Build history of the part. All positions in model axes, mm. Face numbers are marked on the shaded views. A direction names the side the tool comes from. Give positions to 0.01 mm unless a question says otherwise; leave off trailing zeros. Write each loop counter-clockwise with the first axis right and the second up, starting at its lowest first coordinate (ties: lowest second). Pieces come first, ordered by that corner, then holes. Notation, with made-up numbers: (-18, 63) -> (14, 63) arc R19 cw to (14, 89) -> close; hole circle Ø4 at (69, 5.25). An arc over 180 degrees is marked (long way). Put each result on its own line as item: value. Start each with the question number.
Item 1: Slice it at A-A, the plane x = 6.5. List the corners of the cut face in (y, z), plus the area to 3 significant figures.
Item 2: Drill centre lines: line 1 along Y through (x, z) = (0, 10.95); line 2 along Z through (x, y) = (-13, 63.5); line 3 along X through (y, z) = (51.5, -8.25). Where is each one in solid material? Low to high.
Item 3: Slice it at B-B, the plane y = 105. List the corners of the cut face in (x, z).
Item 4: Slice it at D-D, the plane y = 14. List the corners of the cut face in (x, z).
Item 5: Tool access for the marked faces 5 and 6: list every direction of +Z, -Z, +X, -X, +Y, -Y with a clear straight run to the whole face (end or side of a thin tool).
Item 6: Two-plate mould, pull along Z, no slides. Class the marked faces 1, 2, 3 and 4: pulls with the +Z half, pulls with the -Z half, needs draft (parallel to the pull), parting line crosses it, or undercut.
Item 7: Slice it at C-C, the plane z = -0.75. List the corners of the cut face in (x, y), plus the area to 3 significant figures.
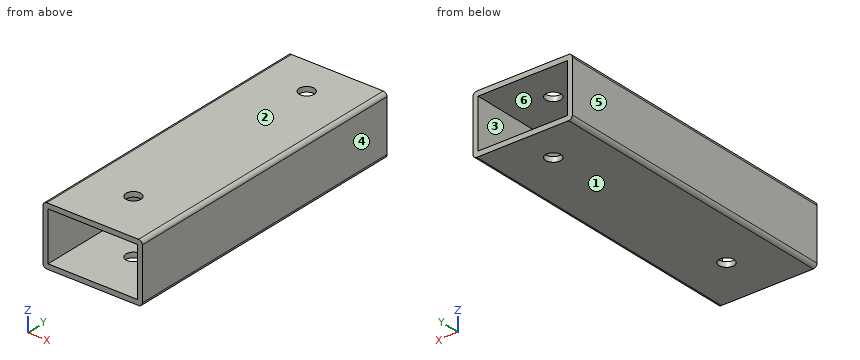
```python
from build123d import *

# Parameters (mm, degrees)
SKETCH1_W               = 39.5
SKETCH1_H               = 23.5
SKETCH1_W_2             = 35.5
SKETCH1_H_2             = 19.5
BOSS_EXTRUDE1_DEPTH     = 120
CUT_EXTRUDE1_DEPTH      = 124.500253036
CUT_EXTRUDE1_DEPTH_BACK = 124.500253036
SKETCH2_R               = 3
FILLET1_R               = 1.5


with BuildPart() as part:
    # Sketch1 → Boss-Extrude1 (new body)
    with BuildSketch(Plane(origin=(0, 0, 0), x_dir=(1, 0, 0), z_dir=(0, 1, 0))):
        Rectangle(SKETCH1_W, SKETCH1_H)
        Rectangle(SKETCH1_W_2, SKETCH1_H_2, mode=Mode.SUBTRACT)
    extrude(amount=BOSS_EXTRUDE1_DEPTH)

    # Sketch2 → Cut-Extrude1 (cut, two sides: drawn at the far end of the back side and taken through both)
    with BuildSketch(Plane(origin=(0, 0, 9.75), x_dir=(-1, 0, 0), z_dir=(0, 0, -1)).offset(-CUT_EXTRUDE1_DEPTH_BACK)):
        with Locations((0, 105)):
            Circle(SKETCH2_R)
        with Locations((0, 20)):
            Circle(SKETCH2_R)
    extrude(amount=CUT_EXTRUDE1_DEPTH + CUT_EXTRUDE1_DEPTH_BACK, mode=Mode.SUBTRACT)

    # Fillet1
    fillet1_edges = [part.edges().sort_by_distance(p)[0] for p in [
        (19.75, 60, 11.75),
        (-19.75, 60, 11.75),
        (-19.75, 60, -11.75),
        (19.75, 60, -11.75),
    ]]
    fillet(fillet1_edges, radius=FILLET1_R)


solid = part.part
```
Values follow:
1. outline: (0, -11.75) -> (120, -11.75) -> (120, -9.75) -> (0, -9.75) -> close; (0, 9.75) -> (120, 9.75) -> (120, 11.75) -> (0, 11.75) -> close
1. area: 480 mm2
2. line 1: 0 to 17, 23 to 102, 108 to 120
2. line 2: -11.75 to -9.75, 9.75 to 11.75
2. line 3: -19.75 to -17.75, 17.75 to 19.75
3. outline: (-19.75, -10.25) arc R1.5 ccw to (-18.25, -11.75) -> (-3, -11.75) -> (-3, -9.75) -> (-17.75, -9.75) -> (-17.75, 9.75) -> (-3, 9.75) -> (-3, 11.75) -> (-18.25, 11.75) arc R1.5 ccw to (-19.75, 10.25) -> close; (3, -11.75) -> (18.25, -11.75) arc R1.5 ccw to (19.75, -10.25) -> (19.75, 10.25) arc R1.5 ccw to (18.25, 11.75) -> (3, 11.75) -> (3, 9.75) -> (17.75, 9.75) -> (17.75, -9.75) -> (3, -9.75) -> close
4. outline: (-19.75, -10.25) arc R1.5 ccw to (-18.25, -11.75) -> (18.25, -11.75) arc R1.5 ccw to (19.75, -10.25) -> (19.75, 10.25) arc R1.5 ccw to (18.25, 11.75) -> (-18.25, 11.75) arc R1.5 ccw to (-19.75, 10.25) -> close; hole (-17.75, -9.75) -> (17.75, -9.75) -> (17.75, 9.75) -> (-17.75, 9.75) -> close
5. face 5: +Z, -Z, -X, +Y, -Y
5. face 6: +Y, -Y
6. face 1: pulls with the -Z half
6. face 2: pulls with the +Z half
6. face 3: undercut
6. face 4: needs draft
7. outline: (-19.75, 0) -> (-17.75, 0) -> (-17.75, 120) -> (-19.75, 120) -> close; (17.75, 0) -> (19.75, 0) -> (19.75, 120) -> (17.75, 120) -> close
7. area: 480 mm2
